```python
from build123d import *

# Parameters (mm, degrees)
SKETCH1_W           = 32
SKETCH1_H           = 8.3
BOSS_EXTRUDE1_DEPTH = 11.2
SKETCH2_W           = 8.3
SKETCH2_H           = 11.2
BOSS_EXTRUDE2_DEPTH = 5
SKETCH3_W           = 8.3
SKETCH3_H           = 11.2
BOSS_EXTRUDE3_DEPTH = 5
FILLET1_R           = 1
FILLET2_R           = 2
SKETCH4_R           = 1.4
CUT_EXTRUDE1_DEPTH  = 8


with BuildPart() as part:
    # Sketch1 → Boss-Extrude1 (new body)
    with BuildSketch(Plane(origin=(0, 0, 0), x_dir=(1, 0, 0), z_dir=(0, 1, 0))):
        Rectangle(SKETCH1_W, SKETCH1_H)
    extrude(amount=BOSS_EXTRUDE1_DEPTH)

    # Sketch2 → Boss-Extrude2 (add)
    with BuildSketch(Plane(origin=(16, 0, 0), x_dir=(0, 0, -1), z_dir=(1, 0, 0))):
        Polygon((-4.15, 11.2), (-16, 11.2), (-16, -4.8), (16, -4.8), (16, 11.2), (4.15, 11.2), (4.15, 0), (-4.15, 0), align=None)
        with Locations((0, 5.6)):
            Rectangle(SKETCH2_W, SKETCH2_H)
    extrude(amount=BOSS_EXTRUDE2_DEPTH)

    # Sketch3 → Boss-Extrude3 (add)
    with BuildSketch(Plane.ZY.offset(16)):
        Polygon((16, 11.2), (4.15, 11.2), (4.15, 0), (-4.15, 0), (-4.15, 11.2), (-16, 11.2), (-16, -4.8), (16, -4.8), align=None)
        with Locations((0, 5.6)):
            Rectangle(SKETCH3_W, SKETCH3_H)
    extrude(amount=BOSS_EXTRUDE3_DEPTH)

    # Fillet1
    fillet1_edges = [part.edges().sort_by_distance(p)[0] for p in [
        (21, 11.2, 0),
        (18.5, 11.2, -16),
        (16, 3.2, 16),
        (18.5, 11.2, 16),
        (21, 3.2, -16),
        (21, 3.2, 16),
        (16, 11.2, -10.075),
        (0, 11.2, 4.15),
        (16, 3.2, -16),
        (16, 11.2, 10.075),
        (-16, 11.2, 10.075),
        (-16, 11.2, -10.075),
        (-18.5, 11.2, 16),
        (-16, 3.2, -16),
        (-18.5, 11.2, -16),
        (-16, 3.2, 16),
        (-21, 11.2, 0),
        (-21, 3.2, -16),
        (-21, 3.2, 16),
        (0, 11.2, -4.15),
    ]]
    fillet(fillet1_edges, radius=FILLET1_R)

    # Fillet2
    fillet2_edges = [part.edges().sort_by_distance(p)[0] for p in [
        (0, 0, 4.15),
        (0, 0, -4.15),
    ]]
    fillet(fillet2_edges, radius=FILLET2_R)

    # Sketch4 → Cut-Extrude1 (cut)
    with BuildSketch(Plane.XZ.offset(4.8)):
        with Locations(Location((-18.5, 0, 0), (0, 0, 270))):
            Circle(SKETCH4_R)
        with Locations(Location((18.5, 0, 0), (0, 0, 270))):
            Circle(SKETCH4_R)
    extrude(amount=-CUT_EXTRUDE1_DEPTH, mode=Mode.SUBTRACT)


solid = part.part
```
Input: part model. Units: mm. Frame: model coordinates. A direction names the side the tool comes from. Round coordinates to 2 decimals unless told otherwise and drop trailing zeros. Loops run counter-clockwise (first coordinate to the right, second up) from the corner with the lowest first, then second, coordinate; pieces in that order, holes last.
1) Section query D-D on y = 8. Return the cut outline in (x, z), plus the area to 3 significant figures.
Ans:
outline: (-21, -15) arc R1 ccw to (-20, -16) - (-17, -16) arc R1 ccw to (-16, -15) - (-16, -4.15) - (16, -4.15) - (16, -15) arc R1 ccw to (17, -16) - (20, -16) arc R1 ccw to (21, -15) - (21, 15) arc R1 ccw to (20, 16) - (17, 16) arc R1 ccw to (16, 15) - (16, 4.15) - (-16, 4.15) - (-16, 15) arc R1 ccw to (-17, 16) - (-20, 16) arc R1 ccw to (-21, 15) - close
area: 584 mm2
2) Section query A-A on z = 7. Return the cut outline in (x, y).
Ans:
outline: (-21, -4.8) - (-16, -4.8) - (-16, 10.2) arc R1 ccw to (-17, 11.2) - (-20, 11.2) arc R1 ccw to (-21, 10.2) - close; (16, -4.8) - (21, -4.8) - (21, 10.2) arc R1 ccw to (20, 11.2) - (17, 11.2) arc R1 ccw to (16, 10.2) - close
3) Pull-direction query (Z, two-part tool) for faces 5 (the cylindrical face through (17.133, -0.856, 0.303)), 6 (the flat face through (-21, 3, 0)), 7 (the cylindrical face through (20.699, 2.805, -15.715)); classes: released by +Z, released by -Z, zero draft, split by the parting line, or undercut.
Ans:
face 5: undercut
face 6: zero draft
face 7: released by -Z
4) Material intervals for line 1 (X direction, y = -2.25, z = 0); line 2 (X direction, y = 5.5, z = -7.5); line 3 (Z direction, x = 2, y = 2.25), sorted ascending.
Ans:
line 1: x = -21 to -19.9, -17.1 to -16, 16 to 17.1, 19.9 to 21
line 2: x = -21 to -16, 16 to 21
line 3: z = -4.15 to 4.15
5) Pin query (flat end, axial travel): pin 1 (4 mm diameter, centred on x = -14.5, y = 4, fed in from -Z); pin 2 (3 mm diameter, centred on x = 15, y = 9, fed in from +Z); pin 3 (2 mm diameter, centred on x = 18.5, z = 0, fed in from -Y). Return the tip coordinate at first contact, or that it passes through.
Ans:
pin 1: stops at z = -15.87
pin 2: stops at z = 15.87
pin 3: stops at y = 3.2
6) Section query B-B on x = 8. Return the cut outline in (y, z), plus the area to 3 significant figures.
Ans:
outline: (0, -2.15) arc R2 ccw to (2, -4.15) - (10.2, -4.15) arc R1 ccw to (11.2, -3.15) - (11.2, 3.15) arc R1 ccw to (10.2, 4.15) - (2, 4.15) arc R2 ccw to (0, 2.15) - close
area: 90.8 mm2
7) Set-up query: faces 1 (the flat face through (0, 6, 4.15)), 2 (the cylindrical face through (-16.301, 10.915, 8.992)), 3 (the flat face through (0, 6, -4.15)), 4 (the cylindrical face through (0.238, 10.915, -3.849)). Return all of +Z, -Z, +X, -X, +Y, -Y with unobstructed straight access to the full face (end or side cutting, diameter ignored); none if empty.
Ans:
face 1: +Z, +Y, -Y
face 2: +Z, +Y
face 3: -Z, +Y, -Y
face 4: -Z, +Y
8) Section query C-C on z = 0. Return the cut outline in (x, y), plus the area to 3 significant figures.
Ans:
outline: (-21, -4.8) - (-19.9, -4.8) - (-19.9, 3.2) - (-17.1, 3.2) - (-17.1, -4.8) - (-16, -4.8) - (-16, 0) - (16, 0) - (16, -4.8) - (17.1, -4.8) - (17.1, 3.2) - (19.9, 3.2) - (19.9, -4.8) - (21, -4.8) - (21, 10.2) arc R1 ccw to (20, 11.2) - (-20, 11.2) arc R1 ccw to (-21, 10.2) - close
area: 473 mm2
